The model under review builds one solid part; all positions refer to its coordinate system, in mm. Coordinates: 2 decimals unless noted, no trailing zeros. Order: outer loops, then holes, each group sorted by start corner. A loop starts at its lowest first (then second) coordinate and runs counter-clockwise, first axis right, second up.
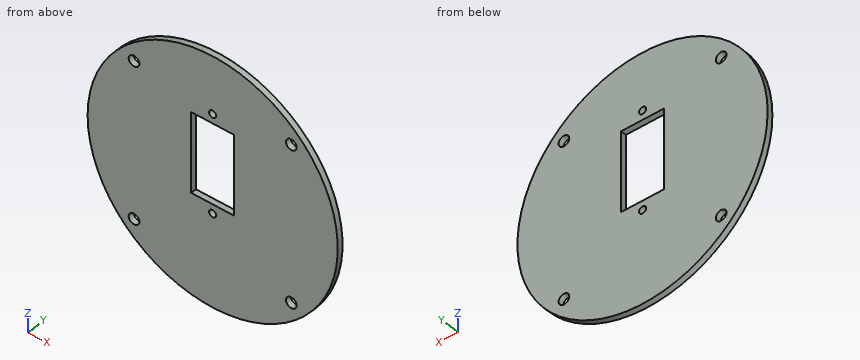
Autodesk Inventor part; units mm, degrees
ref_plane "YZ Plane" through (0, 0, 0) normal (1, 0, 0) x (0, 1, 0)
ref_plane "XZ Plane" through (0, 0, 0) normal (0, 1, 0) x (-1, 0, 0)
ref_plane "XY Plane" through (0, 0, 0) normal (0, 0, 1) x (1, 0, 0)
sketch "Szkic1" plane through (0, 0, 0) normal (0, 1, 0) x (-1, 0, 0)
  circle A0 centre (0, 0) radius 35
  line L0 (-6, -6.25) -> (6, -6.25)
  line L1 (6, -6.25) -> (6, 16.25)
  line L2 (6, 16.25) -> (-6, 16.25)
  line L3 (-6, 16.25) -> (-6, -6.25)
  circle A1 centre (0, 18.85) radius 1
  circle A2 centre (-22, -22) radius 1.5
  circle A3 centre (22, -22) radius 1.5
  circle A4 centre (22, 22) radius 1.5
  circle A5 centre (-22, 22) radius 1.5
  circle A6 centre (0, -8.85) radius 1
  dimension "d0" = 70
  dimension "d1" = 12
  dimension "d2" = 22.5
  dimension "d3" = 2
  dimension "d4" = 2.6
  dimension "d7" = 3
  dimension "d10" = 360
  dimension "d12" = 22
  dimension "d13" = 22
  dimension "d14" = 2
  dimension "d15" = 6
  dimension "d16" = 2.6
  dimension "d17" = 6
  dimension "d18" = 6.25
extrude "Wyciągnięcie proste1" add sketch "Szkic1" along normal blind 1.6
equation "\"d15\" = 0.5 * d1"
equation "\"d17\" = 0.5 * d1"
properties part number "podstawa"
(1) We need section D-D, the plane x = -22. Write out the cut boundary in (y, z), and give its area (3 significant figures).
A:
outline: (0, -27.22) - (1.6, -27.22) - (1.6, -23.5) - (0, -23.5) - close; (0, -20.5) - (1.6, -20.5) - (1.6, 20.5) - (0, 20.5) - close; (0, 23.5) - (1.6, 23.5) - (1.6, 27.22) - (0, 27.22) - close
area: 77.5 mm2
(2) We need section C-C, the plane y = 0.75. Write out the cut boundary in (x, z).
A:
outline: circle Ø70 at (0, 0); hole circle Ø3 at (-22, -22); hole circle Ø3 at (-22, 22); hole (-6, -6.25) - (6, -6.25) - (6, 16.25) - (-6, 16.25) - close; hole circle Ø2 at (0, -8.85); hole circle Ø2 at (0, 18.85); hole circle Ø3 at (22, -22); hole circle Ø3 at (22, 22)
(3) For pin 1 Ø0.5 at (x, y) = (-2.5, 0.5) entering from -Z; pin 2 Ø0.8 at (y, z) = (1, 6) entering from +X; pin 3 Ø0.8 at (x, y) = (2.5, 0.5) entering from +Z, all flat-tipped, find the tip position at first contact; note any pin that passes through.
A:
pin 1: stops at z = -34.93
pin 2: stops at x = 34.55
pin 3: stops at z = 34.94
(4) We need section A-A, the plane z = 0. Write out the cut boundary in (x, y), and give its area (3 significant figures).
A:
outline: (-35, 0) - (-6, 0) - (-6, 1.6) - (-35, 1.6) - close; (6, 0) - (35, 0) - (35, 1.6) - (6, 1.6) - close
area: 92.8 mm2
(5) Wall thickness on probe 1 along Z at (x, y) = (0, 1); probe 2 along X at (y, z) = (1.05, 23); probe 3 along Z at (x, y) = (22, 0.8): over which ranges is each line inside the solid? List them lowest first.
A:
probe 1: z = -35 to -9.85, -7.85 to -6.25, 16.25 to 17.85, 19.85 to 35
probe 2: x = -26.38 to -23.12, -20.88 to 20.88, 23.12 to 26.38
probe 3: z = -27.22 to -23.5, -20.5 to 20.5, 23.5 to 27.22
(6) We need section B-B, the plane x = 0. Write out the cut boundary in (y, z).
A:
outline: (0, -35) - (1.6, -35) - (1.6, -9.85) - (0, -9.85) - close; (0, -7.85) - (1.6, -7.85) - (1.6, -6.25) - (0, -6.25) - close; (0, 16.25) - (1.6, 16.25) - (1.6, 17.85) - (0, 17.85) - close; (0, 19.85) - (1.6, 19.85) - (1.6, 35) - (0, 35) - close
